from build123d import *

# Parameters (mm, degrees)
SKETCH1_R           = 4
SKETCH1_R_2         = 5
BOSS_EXTRUDE1_DEPTH = 8
SKETCH2_R           = 11.5
SKETCH2_R_2         = 1.5
CUT_EXTRUDE1_DEPTH  = 9


with BuildPart() as part:
    # Sketch1 → Boss-Extrude1 (new body)
    with BuildSketch(Plane.XY):
        Polygon((-55.929590299, 11.283196531), (55.49624814, 11.283196531), (55.49624814, -41.637870342), (-55.929590299, -41.637870342), (-55.929590299, -36.557898132), align=None)
        with Locations((38.28332892, -7.416803469)):
            Circle(SKETCH1_R, mode=Mode.SUBTRACT)
        with Locations((-0.21667108, -10.716803469)):
            Circle(SKETCH1_R_2, mode=Mode.SUBTRACT)
        with Locations((-38.71667108, -7.416803469)):
            Circle(SKETCH1_R, mode=Mode.SUBTRACT)
    extrude(amount=BOSS_EXTRUDE1_DEPTH)

    # Sketch2 → Cut-Extrude1 (cut, through all)
    with BuildSketch(Plane.XY.offset(8)):
        with Locations((-0.21667108, -10.716803469)):
            Circle(SKETCH2_R)
        with Locations((-15.71667108, -26.216803469)):
            Circle(SKETCH2_R_2)
        with Locations((15.28332892, -26.216803469)):
            Circle(SKETCH2_R_2)
        with Locations((-15.71667108, 4.783196531)):
            Circle(SKETCH2_R_2)
        with Locations((15.28332892, 4.783196531)):
            Circle(SKETCH2_R_2)
    extrude(amount=-CUT_EXTRUDE1_DEPTH, mode=Mode.SUBTRACT)


solid = part.part
Geometry check sheet. Reference: the model listing, model coordinates, mm. Coordinates: 2 decimals unless noted, no trailing zeros. Order: outer loops, then holes, each group sorted by start corner. A loop starts at its lowest first (then second) coordinate and runs counter-clockwise, first axis right, second up. Notation, with made-up numbers: (23, 13.25) - (28, 13.25) arc R19 ccw to (28, 19.25) - close; hole circle Ø7 at (-40, 42). An arc over 180 degrees is marked (long way). Answer in a Markdown table with one row per item. Add a question column.
1) Cross-section at A-A, the plane y = -13. Record the cut outline in (x, z), then the cut area to 3 significant figures.
2) Release check for a two-part mould opening along Y. For faces 1 (the cylindrical face through (14.093, 3.87, 4.056)), 2 (the flat face through (1, -27, 8)), 3 (the flat face through (1, -41.638, 4)), 4 (the flat face through (-1, 11.283, 4)) record: +Y half, -Y half, draft (parallel to the pull), parting line (faces both ways), or undercut.
3) Cross-section at B-B, the plane x = 2. Record the cut outline in (y, z).
4) Gauge pin test, flat ends, axial feed: P1, Ø4, axis at x = -37.5, y = -17, coming from the -Z side; P2, Ø7, axis at x = -38.72, y = -7.42, coming from the -Z side. Record the tip position at first contact, or that the pin passes through.
5) Material ranges on line 1 along X through (y, z) = (-10.5, 2); line 2 along X through (y, z) = (-8, 4.5); line 3 along Y through (x, z) = (5.5, 7.25), recorded low to high. Write a range as [from, to].
6) Cross-section at C-C, the plane z = 2.75. Record the cut outline in (x, y).
Check result:
| question | item | result |
|---|---|---|
| 1 | outline | (-55.93, 0) - (-11.49, 0) - (-11.49, 8) - (-55.93, 8) - close; (11.05, 0) - (55.5, 0) - (55.5, 8) - (11.05, 8) - close |
| 1 | area | 711 mm² |
| 2 | face 1 | undercut |
| 2 | face 2 | draft |
| 2 | face 3 | -Y half |
| 2 | face 4 | +Y half |
| 3 | outline | (-41.64, 0) - (-22, 0) - (-22, 8) - (-41.64, 8) - close; (0.57, 0) - (11.28, 0) - (11.28, 8) - (0.57, 8) - close |
| 4 | P1 | stops at z = 0 |
| 4 | P2 | passes through |
| 5 | line 1 | x = [-55.93, -41.26], [-36.17, -11.71], [11.28, 35.74], [40.83, 55.5] |
| 5 | line 2 | x = [-55.93, -42.67], [-34.76, -11.39], [10.96, 34.33], [42.24, 55.5] |
| 5 | line 3 | y = [-41.64, -20.7], [-0.74, 11.28] |
| 6 | outline | (-55.93, -41.64) - (55.5, -41.64) - (55.5, 11.28) - (-55.93, 11.28) - close; hole circle Ø8 at (-38.72, -7.42); hole circle Ø3 at (-15.72, -26.22); hole circle Ø3 at (-15.72, 4.78); hole circle Ø23 at (-0.22, -10.72); hole circle Ø3 at (15.28, -26.22); hole circle Ø3 at (15.28, 4.78); hole circle Ø8 at (38.28, -7.42) |
